```python
from build123d import *

# Parameters (mm, degrees)
CONG_1_R                = 0.5
ESQUISSE2_R             = 2.5
ENL_V_MAT_EXTRU_1_DEPTH = 10


with BuildPart() as part:
    # Esquisse1 → Révolution1 (revolve)
    with BuildSketch(Plane(origin=(0, 0, 0), x_dir=(0, 0, -1), z_dir=(1, 0, 0)), mode=Mode.PRIVATE) as r_volution1_sk:
        Polygon((0, 10), (-25, 10), (-25, 0), (-22, 0), (-22, 9), (0, 9), align=None)
    revolve(r_volution1_sk.sketch.rotate(Axis((0, 0, 0), (0, 1, 0)), 180), axis=Axis((0, 0, 0), (0, 1, 0)))

    # Congé1
    cong_1_edges = [part.edges().sort_by_distance(p)[0] for p in [
        (0, 9, 22),
        (0, 10, 25),
    ]]
    fillet(cong_1_edges, radius=CONG_1_R)

    # Esquisse2 → Enlèv. mat.-Extru.1 (cut)
    with BuildSketch(Plane(origin=(0, 10, 0), x_dir=(1, 0, 0), z_dir=(0, 1, 0))):
        with Locations(Location((0, 0, 0), (0, 0, 270))):
            Circle(ESQUISSE2_R)
    extrude(amount=-ENL_V_MAT_EXTRU_1_DEPTH, mode=Mode.SUBTRACT)


solid = part.part
```
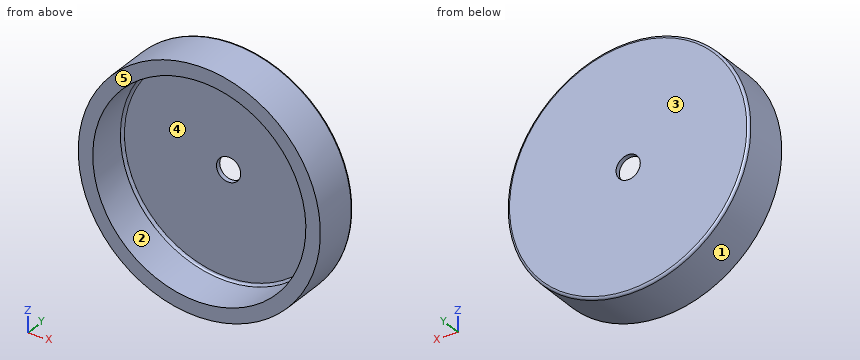
Could you check a few things on this model? Use its own coordinates, in mm. Face numbers are marked on the shaded views. A direction names the side the tool comes from. Coordinates: 2 decimals unless noted, no trailing zeros. Write each loop counter-clockwise with the first axis right and the second up, starting at its lowest first coordinate (ties: lowest second). Pieces come first, ordered by that corner, then holes. Notation, with made-up numbers: (72.25, 39) -> (84.25, 39) arc R31 ccw to (84.25, 63) -> close; hole circle Ø7 at (46.5, -19.75). An arc over 180 degrees is marked (long way). Write item = value, one per line. Start each with the question number.
(1) I want a section at C-C (y = 3.5). Please give me the cut outline in (x, z), plus the area to 3 significant figures.
(2) I want a section at B-B (x = 0). Please give me the cut outline in (y, z).
(3) Will these pins go through, and if not, where does the flat tip stop? pin 1 (2 mm diameter, centred on x = 16, z = 14.5, fed in from -Y); pin 2 (2 mm diameter, centred on y = 1.5, z = 8.5, fed in from -X); pin 3 (1.5 mm diameter, centred on y = 4.5, z = 14.5, fed in from -X); pin 4 (3 mm diameter, centred on x = 0, z = 7.5, fed in from -Y).
(4) Which directions (+Z, -Z, +X, -X, +Y, -Y) give clear straight access to the entire face, cutting with the end or side of a thin tool? Please do the marked faces 4 and 5.
(5) I want a section at A-A (z = 0). Please give me the cut outline in (x, y).
(6) We'd pull the mould along X, two halves only. Please class the marked faces 1, 2 and 3: released by +X, released by -X, zero draft, split by the parting line, or undercut.
(7) I need wall thicknesses on line 1 (X direction, y = 4.5, z = 0); line 2 (X direction, y = 9.3, z = 0); line 3 (Y direction, x = 11.5, z = -9). Which ranges of each line are inside material? Lowest first, please. Write a range as [from, to].
Result set:
q1.outline = circle Ø50 at (0, 0); hole circle Ø44 at (0, 0)
q1.area = 443 mm2
q2.outline = (0, -25) -> (9.5, -25) arc R0.5 ccw to (10, -24.5) -> (10, -2.5) -> (9, -2.5) -> (9, -21.5) arc R0.5 cw to (8.5, -22) -> (0, -22) -> close; (0, 22) -> (8.5, 22) arc R0.5 cw to (9, 21.5) -> (9, 2.5) -> (10, 2.5) -> (10, 24.5) arc R0.5 ccw to (9.5, 25) -> (0, 25) -> close
q3.pin_1 = 0
q3.pin_2 = -23.85
q3.pin_3 = -20.88
q3.pin_4 = 9
q4.face_4 = -Y
q4.face_5 = +Z, -Z, +X, -X, -Y
q5.outline = (-25, 0) -> (-22, 0) -> (-22, 8.5) arc R0.5 cw to (-21.5, 9) -> (-2.5, 9) -> (-2.5, 10) -> (-24.5, 10) arc R0.5 ccw to (-25, 9.5) -> close; (2.5, 9) -> (21.5, 9) arc R0.5 cw to (22, 8.5) -> (22, 0) -> (25, 0) -> (25, 9.5) arc R0.5 ccw to (24.5, 10) -> (2.5, 10) -> close
q6.face_1 = split by the parting line
q6.face_2 = undercut
q6.face_3 = zero draft
q7.line_1 = [-25, -22], [22, 25]
q7.line_2 = [-25, -2.5], [2.5, 25]
q7.line_3 = [9, 10]
